```python
from build123d import *

# Parameters (mm, degrees)
SKETCH2_R           = 12.7
BOSS_EXTRUDE1_DEPTH = 38.1


with BuildPart() as part:
    # Sketch2 → Boss-Extrude1 (new body)
    with BuildSketch(Plane(origin=(0, 0, 0), x_dir=(1, 0, 0), z_dir=(0, 1, 0))):
        with BuildLine():
            Line((0, -38.1), (0, 38.1))
            Line((0, 38.1), (-50.8, 38.1))
            ThreePointArc((-50.8, 38.1), (-43.360512242, 56.060512242), (-25.4, 63.5))
            Line((-25.4, 63.5), (8.89, 63.5))
            ThreePointArc((8.89, 63.5), (34.034717139, 53.084717139), (44.45, 27.94))
            Line((44.45, 27.94), (44.45, -27.94))
            ThreePointArc((44.45, -27.94), (34.034717139, -53.084717139), (8.89, -63.5))
            Line((8.89, -63.5), (-25.4, -63.5))
            ThreePointArc((-25.4, -63.5), (-43.360512242, -56.060512242), (-50.8, -38.1))
            Line((-50.8, -38.1), (0, -38.1))
        make_face()
        with Locations((22.225, 0)):
            Circle(SKETCH2_R, mode=Mode.SUBTRACT)
    extrude(amount=BOSS_EXTRUDE1_DEPTH)


solid = part.part
```
Geometry: final body of the model. Coordinates: model frame, mm. A direction names the side the tool comes from. Round coordinates to 2 decimals unless told otherwise and drop trailing zeros. Order: outer loops, then holes, each group sorted by start corner. A loop starts at its lowest first (then second) coordinate and runs counter-clockwise, first axis right, second up. Notation, with made-up numbers: M -11,70 L 2,70 A27 cw 2,86 Z; hole C -5,-11.75 d7. An arc over 180 degrees is marked long. One line per item, written item: value.
(1) Pull-direction query (Z, two-part tool) for faces 1 (the flat face through (0, 19, 1)), 2 (the cylindrical face through (-43.56, 18.78, -55.86)), 3 (the cylindrical face through (28.085, 18.783, 11.267)), 4 (the flat face through (44.45, 19, 0)); classes: pulls with the +Z half, pulls with the -Z half, needs draft (parallel to the pull), parting line crosses it, or undercut.
Result sheet:
face 1: undercut
face 2: pulls with the -Z half
face 3: undercut
face 4: needs draft
(2) Cut plane A-A (y = 4). Return the cut outline in (x, z) (3 decimals).
Result sheet:
outline: M -50.8,-38.1 A25.4 ccw -25.4,-63.5 L 8.89,-63.5 A35.56 ccw 44.45,-27.94 L 44.45,27.94 A35.56 ccw 8.89,63.5 L -25.4,63.5 A25.4 ccw -50.8,38.1 L 0,38.1 L 0,-38.1 Z; hole C 22.225,0 d25.4
(3) Line query: probe 1 along X at (y, z) = (12, 0) (3 decimals); probe 2 along Z at (x, y) = (-14, 36); probe 3 along X at (y, z) = (10.5, -28.5). Output: solid intervals per line, ascending. Write a range as [from, to].
Result sheet:
probe 1: [0, 9.525], [34.925, 44.45]
probe 2: [-63.5, -38.1], [38.1, 63.5]
probe 3: [0, 44.45]
(4) Cut plane B-B (x = -4). Return the cut outline in (y, z), and give its area (3 significant figures).
Result sheet:
outline: M 0,-63.5 L 38.1,-63.5 L 38.1,-38.1 L 0,-38.1 Z; M 0,38.1 L 38.1,38.1 L 38.1,63.5 L 0,63.5 Z
area: 1,940 mm2
(5) Cut plane C-C (z = 0). Return the cut outline in (x, y) (3 decimals), and give its area (3 significant figures).
Result sheet:
outline: M 0,0 L 9.525,0 L 9.525,38.1 L 0,38.1 Z; M 34.925,0 L 44.45,0 L 44.45,38.1 L 34.925,38.1 Z
area: 726 mm2
(6) Pin query (flat end, axial travel): P1, Ø11.5, axis at x = -32.5, y = 13, coming from the -Z side; P2, Ø6, axis at y = 21, z = -32.5, coming from the +X side; P3, Ø8, axis at y = 32.5, z = -48, coming from the -X side. Return the tip coordinate at first contact, or that it passes through.
Result sheet:
P1: z = -63.46
P2: x = 44.42
P3: x = -50.11
(7) Reachability of faces 5 (the flat face through (-26, 19, 38.1)), 6 (the flat face through (8, 38.1, -1)) from +Z, -Z, +X, -X, +Y, -Y: full face, straight path, thin tool, end or side. Return the list, or none.
Result sheet:
face 5: -X, +Y, -Y
face 6: +Z, -Z, +X, -X, +Y
